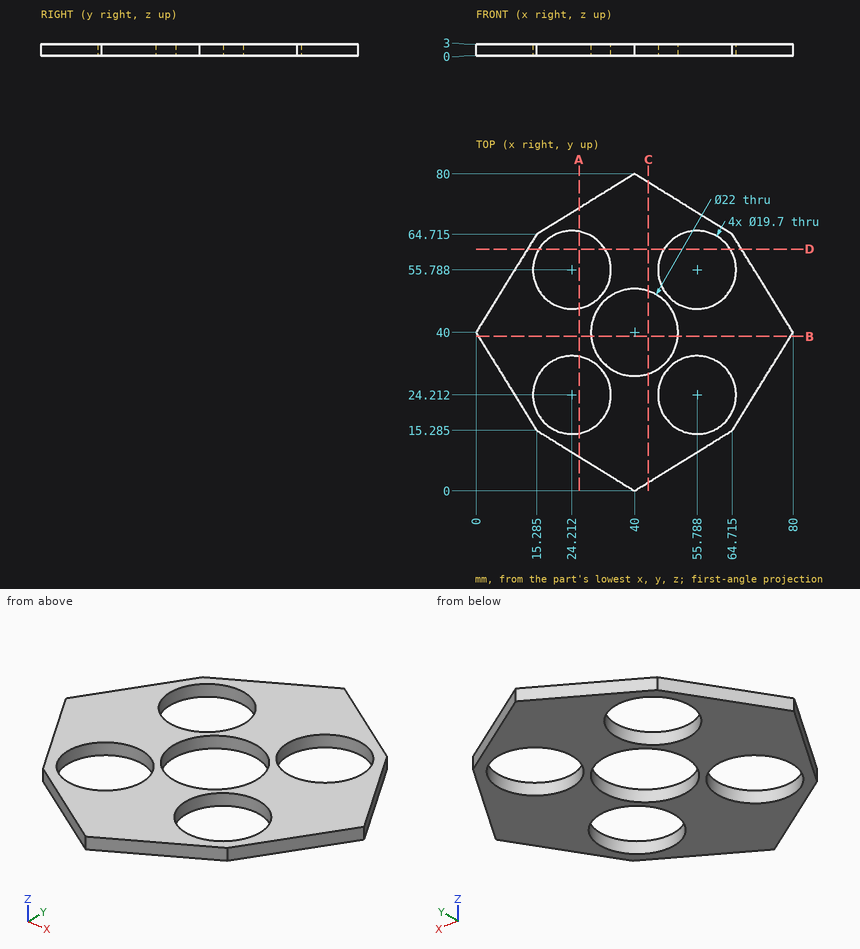
The figure shows three views and two pictorial views of one solid part (mm, origin at its lowest corner). Answer the questions. Give positions to 0.01 mm unless a question says otherwise; leave off trailing zeros. Write each loop counter-clockwise with the first axis right and the second up, starting at its lowest first coordinate (ties: lowest second). Pieces come first, ordered by that corner, then holes. Notation, with made-up numbers: (64, 76.25) -> (115, 76.25) arc R20 cw to (115, 83.25) -> close; hole circle Ø3 at (-11.75, 86.25). An arc over 180 degrees is marked (long way). Answer as a JSON object with one key per item and string values.
1) Section C-C on x = 43.5 is taken. Write down the section's boundary in (y, z) (1 decimal).
Findings below:
{"outline": "(2.2, 0) -> (29.6, 0) -> (29.6, 3) -> (2.2, 3) -> close; (50.4, 0) -> (77.8, 0) -> (77.8, 3) -> (50.4, 3) -> close"}
2) Section A-A on x = 26 is taken. Write down the section's boundary in (y, z).
Findings below:
{"outline": "(8.66, 0) -> (14.53, 0) -> (14.53, 3) -> (8.66, 3) -> close; (33.9, 0) -> (46.1, 0) -> (46.1, 3) -> (33.9, 3) -> close; (65.47, 0) -> (71.34, 0) -> (71.34, 3) -> (65.47, 3) -> close"}
3) Flat-ended cylindrical pins translate along their axes: pin 1 Ø13 at (x, y) = (40, 40) entering from -Z; pin 2 Ø1.5 at (x, z) = (23, 0.5) entering from +Y; pin 3 Ø1 at (x, z) = (15.5, 2.5) entering from +Y. Find the tip coordinate at first contact, or state that the pin passes through.
Findings below:
{"pin 1": "passes through", "pin 2": "stops at y = 69.95", "pin 3": "stops at y = 65.16"}
4) Section D-D on y = 61 is taken. Write down the section's boundary in (x, z) (1 decimal).
Findings below:
{"outline": "(13, 0) -> (15.9, 0) -> (15.9, 3) -> (13, 3) -> close; (32.6, 0) -> (47.4, 0) -> (47.4, 3) -> (32.6, 3) -> close; (64.1, 0) -> (67, 0) -> (67, 3) -> (64.1, 3) -> close"}
5) Section B-B on y = 39 is taken. Write down the section's boundary in (x, z) (1 decimal).
Findings below:
{"outline": "(0.6, 0) -> (29, 0) -> (29, 3) -> (0.6, 3) -> close; (51, 0) -> (79.4, 0) -> (79.4, 3) -> (51, 3) -> close"}
6) Straight lines are drawn through the part: probe 1 along Y at (x, z) = (52, 2.3) (1 decimal); probe 2 along X at (y, z) = (54.5, 0.85); probe 3 along X at (y, z) = (63.5, 1.3) (1 decimal). For each, find the intervals that lie inside material, in ascending order. Write a range as from..to.
Findings below:
{"probe 1": "y = 7.4..15.1, 33.3..46.7, 64.9..72.6", "probe 2": "x = 8.97..14.45, 33.98..46.02, 65.55..71.03", "probe 3": "x = 14.5..18.1, 30.3..49.7, 61.9..65.5"}
